For this review, take the finished solid that the model builds, in its own axes (mm). A direction names the side the tool comes from. Coordinates: 2 decimals unless noted, no trailing zeros. Loops run counter-clockwise (first coordinate to the right, second up) from the corner with the lowest first, then second, coordinate; pieces in that order, holes last. Notation, with made-up numbers: M 39.5,-10 L 56.5,-10 A23 cw 56.5,20 Z; hole C -15.75,-32 d2. An arc over 180 degrees is marked long. Answer as a JSON object with one key per item and string values. Group by question number.
Item 1: Tool access review of faces 1 (the face through (-55, -25, 33.773)), 2 (the face through (-13, -15, 50.8)), 3 (the face through (-28, 0, 26)): name each direction out of +Z, -Z, +X, -X, +Y, -Y from which nothing blocks a thin tool from reaching the whole face with its end or side.
Item 2: Add section A-A (z = 25.4). State the section outline as (x, y) points.
Item 3: Add section C-C (x = 14). State the section outline as (y, z) points, then the cut area to 3 significant figures.
Item 4: Mouldability with a two-part tool opening along X and no side actions: class faces 4 (the face through (-52.658, -25, 26)), 5 (the face through (-102.64, -25.04, 26.8)), 6 (the face through (39.47, -14.88, 30.17)), 7 (the face through (-14, -15, 0)) as +X half, -X half, draft (parallel to the pull), parting line (faces both ways), or undercut.
Item 5: Wall thickness on L1, parallel to X at y = -12, z = 25; L2, parallel to X at y = -5.5, z = 38.5; L3, parallel to Z at x = -10, y = -15: over which ranges is each line inside the solid? List them lowest first. Write a range as from..to.
Item 6: Insertion check: pin 1 (10 mm diameter, centred on x = -81.5, y = -44, fed in from -Z); pin 2 (9 mm diameter, centred on x = -22, y = -11.5, fed in from -Z); pin 3 (5 mm diameter, centred on x = -34, z = 48.5, fed in from -Y). Each pin has a flat end and moves straight along its axis. Give the tip position at first contact, or say it passes through.
Item 7: Add section B-B (y = -25.5). State the section outline as (x, z) points (3 decimals), then the cut area to 3 significant figures.
Item 8: Add section D-D (y = -39.5). State the section outline as (x, z) points (3 decimals), then the cut area to 3 significant figures.
from build123d import *

# Parameters (mm, degrees)
F0_R     = 15.875
F1_DEPTH = 30.1752
F2_R     = 31.75
F3_DEPTH = 50.8


with BuildPart() as f1:
    # F0 (on Front) → F1 (new body)
    with BuildSketch(Plane.XZ):
        with BuildLine():
            ThreePointArc((-39.171085, 25.4), (-42.523022, 11.200968), (-51.871085, 0))
            Line((-51.871085, 0), (24.328915, 0))
            ThreePointArc((24.328915, 0), (49.728915, 25.4), (24.328915, 50.8))
            Line((24.328915, 50.8), (-51.871085, 50.8))
            ThreePointArc((-51.871085, 50.8), (-42.523022, 39.599032), (-39.171085, 25.4))
        make_face()
        with Locations((24.328915, 25.4)):
            Circle(F0_R, mode=Mode.SUBTRACT)
    extrude(amount=F1_DEPTH)

    # F2 (on Front) → F3 (join)
    with BuildSketch(Plane.XZ):
        with Locations((-70.921085, 25.4)):
            Circle(F2_R)
        with BuildLine():
            ThreePointArc((-57.433685, 17.027087), (-86.796085, 25.4), (-57.433685, 33.772913))
            Line((-57.433685, 33.772913), (-52.658485, 33.772913))
            Line((-52.658485, 33.772913), (-52.658485, 17.027087))
            Line((-52.658485, 17.027087), (-57.433685, 17.027087))
        make_face(mode=Mode.SUBTRACT)
    extrude(amount=F3_DEPTH)


solid = f1.part
From the geometry:
{
 "1": {"face 1": "+Y, -Y", "face 2": "+Z, +X, +Y, -Y", "face 3": "+Z, -Z, +X, -X, +Y"},
 "2": {"outline": "M -102.67,-50.8 L -86.8,-50.8 L -86.8,0 L -102.67,0 Z; M -52.66,-50.8 L -39.17,-50.8 L -39.17,-30.18 L 8.45,-30.18 L 8.45,0 L -52.66,0 Z; M 40.2,-30.18 L 49.73,-30.18 L 49.73,0 L 40.2,0 Z"},
 "3": {"outline": "M -30.18,0 L 0,0 L 0,13.34 L -30.18,13.34 Z; M -30.18,37.46 L 0,37.46 L 0,50.8 L -30.18,50.8 Z", "area": "805 mm²"},
 "4": {"face 4": "undercut", "face 5": "parting line", "face 6": "undercut", "face 7": "draft"},
 "5": {"L1": "x = -102.67..-86.79, -52.66..8.46, 40.2..49.73", "L2": "x = -99.84..-79.89, -61.95..15.36, 33.3..46.09", "L3": "z = 0..50.8"},
 "6": {"pin 1": "stops at z = -5.86", "pin 2": "stops at z = 0", "pin 3": "stops at y = -30.18"},
 "7": {"outline": "M -51.871,0 L 24.329,0 A25.4 ccw 24.329,50.8 L -51.871,50.8 A31.75 ccw long Z; hole M -57.434,17.027 L -52.658,17.027 L -52.658,33.773 L -57.434,33.773 A15.875 ccw long Z; hole C 24.329,25.4 d31.75", "area": "5,960 mm²"},
 "8": {"outline": "C -70.921,25.4 d63.5; hole M -57.434,17.027 L -52.658,17.027 L -52.658,33.773 L -57.434,33.773 A15.875 ccw long Z", "area": "2,320 mm²"}
}
